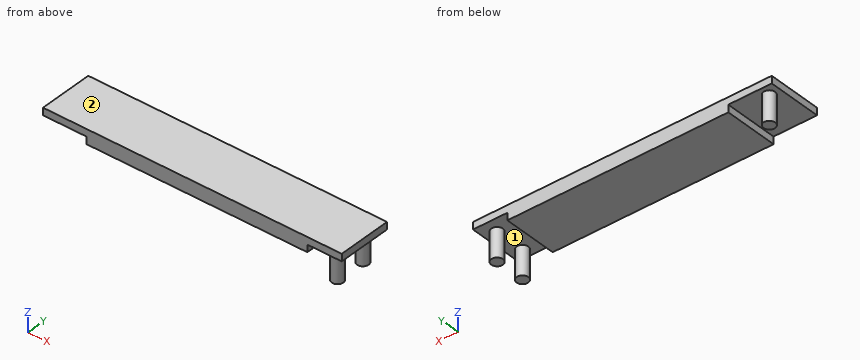
```python
from build123d import *

# Parameters (mm, degrees)
CYLINDER_R        = 1.6
CYLINDER_DEPTH    = 10
BOX001_W          = 61
BOX001_H          = 15
BOX001_DEPTH      = 2
BOX_W             = 82.5
BOX_H             = 15
BOX_DEPTH         = 2
CYLINDER003_R     = 1.6
CYLINDER003_DEPTH = 10
CYLINDER002_R     = 1.6
CYLINDER002_DEPTH = 10


with BuildPart() as taladro1:
    # Cylinder → Cylinder (new body)
    with BuildSketch(Plane(origin=(0, 1.2, -10), x_dir=(1, 0, 0), z_dir=(0, 0, 1))):
        Circle(CYLINDER_R)
    extrude(amount=CYLINDER_DEPTH)


with BuildPart() as perfora_2mm_centro:
    # Box001 → Box001 (new body)
    with BuildSketch(Plane(origin=(12, 0, -2), x_dir=(1, 0, 0), z_dir=(0, 0, 1))):
        with Locations((30.5, 7.5)):
            Rectangle(BOX001_W, BOX001_H)
    extrude(amount=BOX001_DEPTH)


with BuildPart() as fusion001:
    # Box → Box (new body)
    with BuildSketch(Plane.XY):
        with Locations((41.25, 7.5)):
            Rectangle(BOX_W, BOX_H)
    extrude(amount=BOX_DEPTH)

    # Fusion: union perfora_2mm_centro
    add(perfora_2mm_centro.part)


with BuildPart() as fusion001_1:
    # Fusion placement: moved
    add(fusion001.part.moved(Location((-3, -11, -2))))

    # Fusion001: union taladro1
    add(taladro1.part)


with BuildPart() as fusion002:
    # Cylinder003 → Cylinder003 (new body)
    with BuildSketch(Plane(origin=(76, 0.2, -10), x_dir=(1, 0, 0), z_dir=(0, 0, 1))):
        Circle(CYLINDER003_R)
    extrude(amount=CYLINDER003_DEPTH)

    # Fusion002: union Fusion001
    add(fusion001_1.part)


with BuildPart() as fusion007:
    # Cylinder002 → Cylinder002 (new body)
    with BuildSketch(Plane(origin=(76, -8.2, -10), x_dir=(1, 0, 0), z_dir=(0, 0, 1))):
        Circle(CYLINDER002_R)
    extrude(amount=CYLINDER002_DEPTH)

    # Fusion007: union Fusion002
    add(fusion002.part)


solid = fusion007.part
```
The model under review builds one solid part; all positions refer to its coordinate system, in mm. Face numbers are marked on the shaded views. Round coordinates to 2 decimals unless told otherwise and drop trailing zeros. Order: outer loops, then holes, each group sorted by start corner. A loop starts at its lowest first (then second) coordinate and runs counter-clockwise, first axis right, second up.
(1) Mouldability with a two-part tool opening along X and no side actions: class the marked faces 1 and 2 as released by +X, released by -X, zero draft, split by the parting line, or undercut.
Working result:
face 1: undercut
face 2: zero draft
(2) Take a section at B-B, the plane y = -3.25. State the section outline as (x, z) points, plus the area to 3 significant figures.
Working result:
outline: (-3, -2) - (9, -2) - (9, -4) - (70, -4) - (70, -2) - (79.5, -2) - (79.5, 0) - (-3, 0) - close
area: 287 mm2
(3) Take a section at A-A, the plane x = 76. State the section outline as (y, z) points, plus the area to 3 significant figures.
Working result:
outline: (-11, -2) - (-9.8, -2) - (-9.8, -10) - (-6.6, -10) - (-6.6, -2) - (-1.4, -2) - (-1.4, -10) - (1.8, -10) - (1.8, -2) - (4, -2) - (4, 0) - (-11, 0) - close
area: 81.2 mm2
(4) Wall thickness on L1, parallel to Z at x = 39.5, y = 3.25; L2, parallel to X at y = -0.5, z = -2.25; L3, parallel to Z at x = 7, y = -2.75: over which ranges is each line inside the solid? List them lowest first.
Working result:
L1: z = -4 to 0
L2: x = 9 to 70, 74.56 to 77.44
L3: z = -2 to 0
(5) Take a section at D-D, the plane x = 0. State the section outline as (y, z) points, plus the area to 3 significant figures.
Working result:
outline: (-11, -2) - (-0.4, -2) - (-0.4, -10) - (2.8, -10) - (2.8, -2) - (4, -2) - (4, 0) - (-11, 0) - close
area: 55.6 mm2
(6) Take a section at C-C, the plane z = -6.25. State the section outline as (x, y) points.
Working result:
outline: circle Ø3.2 at (0, 1.2); circle Ø3.2 at (76, -8.2); circle Ø3.2 at (76, 0.2)
(7) For P1, Ø0.6, axis at y = -3, z = -3, coming from the +X side; P2, Ø7.5, axis at x = 72.5, y = -3.5, coming from the -Z side; P3, Ø6, axis at x = 1, y = -4, coming from the -Z side; P4, Ø4.5, axis at x = 25.5, y = -3.5, coming from the -Z side, all flat-tipped, find the tip position at first contact; note any pin that passes through.
Working result:
P1: stops at x = 70
P2: stops at z = -10
P3: stops at z = -2
P4: stops at z = -4
